Verification items for the finished model (mm, model axes). Face numbers are marked on the shaded views. Give positions to 0.01 mm unless a question says otherwise; leave off trailing zeros. Loops run counter-clockwise (first coordinate to the right, second up) from the corner with the lowest first, then second, coordinate; pieces in that order, holes last. Notation, with made-up numbers: M 72,-3.5 L 100,-3.5 A22 cw 100,35.5 Z; hole C -2,7 d9. An arc over 180 degrees is marked long. Use a Markdown table: item, result.
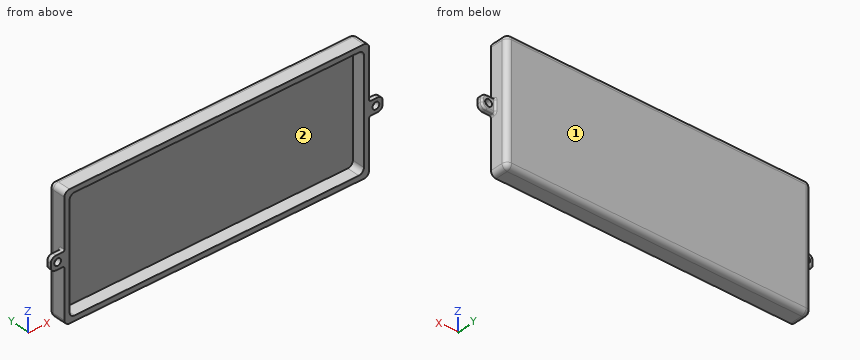
from build123d import *

# Parameters (mm, degrees)
SKETCH1_W           = 179
SKETCH1_H           = 72
BOSS_EXTRUDE1_DEPTH = 10.5
SHELL1_T            = -3
SKETCH2_W           = 8
SKETCH2_H           = 3
BOSS_EXTRUDE2_DEPTH = 8
SKETCH3_W           = 8
SKETCH3_H           = 3
BOSS_EXTRUDE3_DEPTH = 8
SKETCH4_R           = 2
CUT_EXTRUDE1_DEPTH  = 8
SKETCH5_R           = 2
CUT_EXTRUDE2_DEPTH  = 8
FILLET1_R           = 3
FILLET2_R           = 1


with BuildPart() as part:
    # Sketch1 → Boss-Extrude1 (new body)
    with BuildSketch(Plane(origin=(0, 0, 0), x_dir=(1, 0, 0), z_dir=(0, 1, 0))):
        Rectangle(SKETCH1_W, SKETCH1_H)
    extrude(amount=BOSS_EXTRUDE1_DEPTH)

    # Shell1
    shell1_openings = [part.faces().sort_by_distance(p)[0] for p in [
        (0, 0, 0),
    ]]
    offset(amount=SHELL1_T, openings=shell1_openings, kind=Kind.INTERSECTION)

    # Sketch2 → Boss-Extrude2 (add)
    with BuildSketch(Plane.ZY.offset(89.5)):
        with Locations((0, 1.5)):
            Rectangle(SKETCH2_W, SKETCH2_H)
    extrude(amount=BOSS_EXTRUDE2_DEPTH)

    # Sketch3 → Boss-Extrude3 (add)
    with BuildSketch(Plane(origin=(89.5, 0, 0), x_dir=(0, 0, -1), z_dir=(1, 0, 0))):
        with Locations((0, 1.5)):
            Rectangle(SKETCH3_W, SKETCH3_H)
    extrude(amount=BOSS_EXTRUDE3_DEPTH)

    # Sketch4 → Cut-Extrude1 (cut)
    with BuildSketch(Plane(origin=(0, 3, 0), x_dir=(1, 0, 0), z_dir=(0, 1, 0))):
        with Locations(Location((-93.5, 0, 0), (0, 0, 270))):
            Circle(SKETCH4_R)
    extrude(amount=-CUT_EXTRUDE1_DEPTH, mode=Mode.SUBTRACT)

    # Sketch5 → Cut-Extrude2 (cut)
    with BuildSketch(Plane(origin=(0, 3, 0), x_dir=(1, 0, 0), z_dir=(0, 1, 0))):
        with Locations(Location((93.5, 0, 0), (0, 0, 270))):
            Circle(SKETCH5_R)
    extrude(amount=-CUT_EXTRUDE2_DEPTH, mode=Mode.SUBTRACT)

    # Fillet1
    fillet1_edges = [part.edges().sort_by_distance(p)[0] for p in [
        (-89.5, 10.5, 0),
        (86.5, 3.75, 33),
        (86.5, 3.75, -33),
        (-86.5, 3.75, -33),
        (-86.5, 3.75, 33),
        (0, 10.5, 36),
        (-97.5, 1.5, -4),
        (-97.5, 1.5, 4),
        (97.5, 1.5, 4),
        (97.5, 1.5, -4),
        (89.5, 10.5, 0),
        (89.5, 5.25, 36),
        (-89.5, 5.25, 36),
        (-89.5, 5.25, -36),
        (89.5, 5.25, -36),
        (0, 10.5, -36),
    ]]
    fillet(fillet1_edges, radius=FILLET1_R)

    # Fillet2
    fillet2_edges = [part.edges().sort_by_distance(p)[0] for p in [
        (92, 3, -4),
        (96.621320344, 3, -3.121320344),
        (96.621320344, 3, 3.121320344),
        (-97.5, 3, 0),
        (-92, 3, -4),
        (-92, 3, 4),
        (-96.621320344, 3, 3.121320344),
        (-96.621320344, 3, -3.121320344),
        (-89.5, 1.5, -4),
        (-89.5, 1.5, 4),
        (-89.5, 3, 0),
        (89.5, 1.5, 4),
        (89.5, 1.5, -4),
        (89.5, 3, 0),
        (97.5, 3, 0),
        (92, 3, 4),
    ]]
    fillet(fillet2_edges, radius=FILLET2_R)


solid = part.part
(1) Draft check along X on the marked faces 1 and 2. Enter one of: +X half, -X half, draft (parallel to the pull), parting line (faces both ways), or undercut.
Results below:
| item | result |
|---|---|
| face 1 | draft |
| face 2 | undercut |
(2) Gauge pin test, flat ends, axial feed: P1, Ø0.6, axis at x = -92, y = 1, coming from the +Z side; P2, Ø0.6, axis at x = 92.5, y = 0.5, coming from the -Z side; P3, Ø3, axis at y = 3.5, z = -6.5, coming from the -X side. Record the tip position at first contact, or that the pin passes through.
Results below:
| item | result |
|---|---|
| P1 | z = 4 |
| P2 | z = -4 |
| P3 | x = -89.5 |
(3) Cross-section at C-C on z = -26. Record the cut outline in (x, y).
Results below:
| item | result |
|---|---|
| outline | M -89.5,0 L -86.5,0 L -86.5,7.5 L 86.5,7.5 L 86.5,0 L 89.5,0 L 89.5,7.5 A3 ccw 86.5,10.5 L -86.5,10.5 A3 ccw -89.5,7.5 Z |
(4) Cross-section at A-A on y = 5.75. Record the cut outline in (x, z), then the cut area to 3 significant figures.
Results below:
| item | result |
|---|---|
| outline | M -89.5,-33 A3 ccw -86.5,-36 L 86.5,-36 A3 ccw 89.5,-33 L 89.5,33 A3 ccw 86.5,36 L -86.5,36 A3 ccw -89.5,33 Z; hole M -86.5,-30 A3 ccw -83.5,-33 L 83.5,-33 A3 ccw 86.5,-30 L 86.5,30 A3 ccw 83.5,33 L -83.5,33 A3 ccw -86.5,30 Z |
| area | 1,470 mm^2 |
(5) Material ranges on line 1 (X direction, y = 2.25, z = 0); line 2 (X direction, y = 4, z = 8); line 3 (X direction, y = 2.35, z = 0), recorded low to high.
Results below:
| item | result |
|---|---|
| line 1 | -97.47 to -95.5, -91.5 to -86.5, 86.5 to 91.5, 95.5 to 97.47 |
| line 2 | -89.5 to -86.5, 86.5 to 89.5 |
| line 3 | -97.44 to -95.5, -91.5 to -86.5, 86.5 to 91.5, 95.5 to 97.44 |
(6) Cross-section at B-B on x = -18.5. Record the cut outline in (y, z), then the cut area to 3 significant figures.
Results below:
| item | result |
|---|---|
| outline | M 0,-36 L 7.5,-36 A3 ccw 10.5,-33 L 10.5,33 A3 ccw 7.5,36 L 0,36 L 0,33 L 7.5,33 L 7.5,-33 L 0,-33 Z |
| area | 257 mm^2 |
